```python
from build123d import *

# Parameters (mm, degrees)
BOSS_EXTRUDE1_DEPTH = 5
BOSS_EXTRUDE2_DEPTH = 15
SKETCH4_R           = 1.75
CUT_EXTRUDE1_DEPTH  = 5
FILLET2_R           = 2


with BuildPart() as part:
    # Sketch1 → Boss-Extrude1 (new body)
    with BuildSketch(Plane.XY):
        with BuildLine():
            Line((-68.75, 0), (68.75, 0))
            Line((68.75, 0), (68.75, 4))
            Line((68.75, 4), (48.75, 4))
            Line((48.75, 4), (32.109157698, 86.934581855))
            ThreePointArc((32.109157698, 86.934581855), (25.174943055, 98.470805362), (12.5, 103))
            Line((12.5, 103), (-12.5, 103))
            ThreePointArc((-12.5, 103), (-25.174943055, 98.470805362), (-32.109157698, 86.934581855))
            Line((-32.109157698, 86.934581855), (-48.75, 4))
            Line((-48.75, 4), (-68.75, 4))
            Line((-68.75, 4), (-68.75, 0))
        make_face()
        with BuildLine():
            Line((-12.5, 98), (12.5, 98))
            ThreePointArc((12.5, 98), (14.5, 96), (12.5, 94))
            Line((12.5, 94), (-12.5, 94))
            ThreePointArc((-12.5, 94), (-14.5, 96), (-12.5, 98))
        make_face(mode=Mode.SUBTRACT)
        with BuildLine():
            Line((-12.5, 89), (12.5, 89))
            ThreePointArc((12.5, 89), (26, 75.5), (12.5, 62))
            Line((12.5, 62), (-12.5, 62))
            ThreePointArc((-12.5, 62), (-26, 75.5), (-12.5, 89))
        make_face(mode=Mode.SUBTRACT)
        with BuildLine():
            Line((-12.5, 57), (12.5, 57))
            ThreePointArc((12.5, 57), (14.5, 55), (12.5, 53))
            Line((12.5, 53), (-12.5, 53))
            ThreePointArc((-12.5, 53), (-14.5, 55), (-12.5, 57))
        make_face(mode=Mode.SUBTRACT)
    extrude(amount=BOSS_EXTRUDE1_DEPTH)

    # Sketch2 → Boss-Extrude2 (add)
    with BuildSketch(Plane.XY.offset(5)):
        Polygon((-39.620414876, 49.5), (39.620414876, 49.5), (48.75, 4), (68.75, 4), (68.75, 0), (-68.75, 0), (-68.75, 4), (-48.75, 4), align=None)
        Polygon((-35.524007883, 44.5), (-43.449691672, 5), (43.449691672, 5), (35.524007883, 44.5), align=None, mode=Mode.SUBTRACT)
    extrude(amount=BOSS_EXTRUDE2_DEPTH)

    # Sketch4 → Cut-Extrude1 (cut, through all)
    with BuildSketch(Plane(origin=(0, 4, 0), x_dir=(1, 0, 0), z_dir=(0, 1, 0))):
        with Locations((-58.75, -10)):
            Circle(SKETCH4_R)
        with Locations((58.75, -10)):
            Circle(SKETCH4_R)
    extrude(amount=-CUT_EXTRUDE1_DEPTH, mode=Mode.SUBTRACT)

    # Fillet2
    fillet2_edges = [part.edges().sort_by_distance(p)[0] for p in [
        (68.75, 2, 0),
        (-68.75, 2, 0),
        (-68.75, 2, 20),
        (68.75, 2, 20),
    ]]
    fillet(fillet2_edges, radius=FILLET2_R)


solid = part.part
```
Read the model definition and answer for the solid it produces. Units are mm, in the model's axes. A direction names the side the tool comes from. Round coordinates to 2 decimals unless told otherwise and drop trailing zeros. Loops run counter-clockwise (first coordinate to the right, second up) from the corner with the lowest first, then second, coordinate; pieces in that order, holes last. Notation, with made-up numbers: (18.5, -14) -> (74.5, -14) arc R8 cw to (74.5, -8) -> close; hole circle Ø11 at (45.5, -36.5). An arc over 180 degrees is marked (long way). One line per item, written item: value.
1) Flat-ended cylindrical pins translate along their axes: P1, Ø3, axis at x = -58.75, z = 10, coming from the -Y side; P2, Ø8, axis at x = 16, z = 3.5, coming from the +Y side; P3, Ø4, axis at y = 45, z = 12.5, coming from the +X side; P4, Ø4, axis at y = 32.5, z = 11.5, coming from the -X side. Find the tip coordinate at first contact, or state that the pin passes through.
Answer list:
P1: passes through
P2: stops at y = 103
P3: stops at x = 40.92
P4: stops at x = -43.43
2) A cutting plane is placed at D-D (y = 42). Determine the outline of the cut face in (x, z).
Answer list:
outline: (-41.13, 0) -> (41.13, 0) -> (41.13, 20) -> (36.03, 20) -> (36.03, 5) -> (-36.03, 5) -> (-36.03, 20) -> (-41.13, 20) -> close
3) A cutting plane is placed at A-A (z = 10). Determine the outline of the cut face in (x, y).
Answer list:
outline: (-68.75, 0) -> (-60.5, 0) -> (-60.5, 4) -> (-68.75, 4) -> close; (-57, 0) -> (57, 0) -> (57, 4) -> (48.75, 4) -> (39.62, 49.5) -> (-39.62, 49.5) -> (-48.75, 4) -> (-57, 4) -> close; (60.5, 0) -> (68.75, 0) -> (68.75, 4) -> (60.5, 4) -> close; hole (-43.45, 5) -> (43.45, 5) -> (35.52, 44.5) -> (-35.52, 44.5) -> close
4) For faces 4 (the face through (61, 4, 10)), 5 (the face through (-1, 49.5, 12)), 6 (the face through (0.3, 4.7, 20)), 7 (the face through (-1, 25, 5)), 8 (the face through (14.5, 96, 2.5)), determine the directions among +Z, -Z, +X, -X, +Y, -Y from which every point of the face is accessible in a straight line to the end or side of a thin tool.
Answer list:
face 4: +Z, -Z, +X, +Y
face 5: +Z, +X, -X, +Y
face 6: +Z, +X, -X, +Y, -Y
face 7: +Z
face 8: +Z, -Z
5) Consider L1, parallel to X at y = 1.65, z = 10; L2, parallel to Z at x = 58.75, y = 1.2; L3, parallel to Y at x = 6.5, z = 19. Determine where each line is inside the solid, lowest interval first. Write a range as [from, to].
Answer list:
L1: x = [-68.75, -60.5], [-57, 57], [60.5, 68.75]
L2: z = [0, 8.25], [11.75, 20]
L3: y = [0, 5], [44.5, 49.5]
6) A cutting plane is placed at B-B (x = -58.75). Determine the outline of the cut face in (y, z).
Answer list:
outline: (0, 0) -> (4, 0) -> (4, 8.25) -> (0, 8.25) -> close; (0, 11.75) -> (4, 11.75) -> (4, 20) -> (0, 20) -> close
7) A cutting plane is placed at C-C (y = 96). Determine the outline of the cut face in (x, z), and give its area (3 significant figures).
Answer list:
outline: (-27.7, 0) -> (-14.5, 0) -> (-14.5, 5) -> (-27.7, 5) -> close; (14.5, 0) -> (27.7, 0) -> (27.7, 5) -> (14.5, 5) -> close
area: 132 mm²
8) The mould has two halves that part along Y. Classify faces 1 (the face through (-57.081, 2.028, 9.474)), 2 (the face through (1, 0, 10)), 3 (the face through (-1, 5, 12)): pulls with the +Y half, pulls with the -Y half, needs draft (parallel to the pull), parting line crosses it, or undercut.
Answer list:
face 1: needs draft
face 2: pulls with the -Y half
face 3: undercut
